```python
from build123d import *

# Parameters (mm, degrees)
BOSS_EXTRUDE1_DEPTH = 11.1125
SKETCH2_R           = 3.96875
BOSS_EXTRUDE2_DEPTH = 9.525
SKETCH4_R           = 3.96875
BOSS_EXTRUDE3_DEPTH = 9.525
FILLET1_R           = 3.175


with BuildPart() as part:
    # Sketch1 → Boss-Extrude1 (new body)
    with BuildSketch(Plane(origin=(0, 0, 0), x_dir=(1, 0, 0), z_dir=(0, 1, 0))):
        with BuildLine():
            Line((-6.133628997, -1.643500936), (-18.005791029, 42.664010964))
            Line((-18.005791029, 42.664010964), (-17.239087405, 42.869448581))
            Line((-17.239087405, 42.869448581), (-5.366925372, -1.438063319))
            ThreePointArc((-5.366925372, -1.438063319), (0.484259096, -5.535106791), (5.535106791, -0.484259096))
            Line((5.535106791, -0.484259096), (9.532985307, 45.211701443))
            Line((9.532985307, 45.211701443), (10.323714849, 45.142521572))
            Line((10.323714849, 45.142521572), (6.325836333, -0.553438966))
            ThreePointArc((6.325836333, -0.553438966), (0.553438966, -6.325836333), (-6.133628997, -1.643500936))
        make_face()
    extrude(amount=BOSS_EXTRUDE1_DEPTH)

    # Sketch2 → Boss-Extrude2 (add)
    with BuildSketch(Plane(origin=(6.325836333, 0, 0.553438966), x_dir=(0.08715574274765789, 0, -0.9961946980917457), z_dir=(0.9961946980917457, 0, 0.08715574274765789))):
        with Locations(Location((39.520511684, 5.55625, 0), (0, 0, 180))):
            Circle(SKETCH2_R)
    extrude(amount=BOSS_EXTRUDE2_DEPTH)

    # Sketch4 → Boss-Extrude3 (add)
    with BuildSketch(Plane(origin=(-6.133628997, 0, 1.643500936), x_dir=(0.2588190451025218, 0, 0.9659258262890681), z_dir=(-0.9659258262890681, 0, 0.2588190451025218))):
        with Locations((-39.520511684, 5.55625)):
            Circle(SKETCH4_R)
    extrude(amount=BOSS_EXTRUDE3_DEPTH)

    # Fillet1
    fillet1_edges = [part.edges().sort_by_distance(p)[0] for p in [
        (19.604929736, 5.55625, -41.940174498),
        (-26.589921674, 5.55625, -37.898648686),
    ]]
    fillet(fillet1_edges, radius=FILLET1_R)


solid = part.part
```
Verification items for the finished model (mm, model axes). A direction names the side the tool comes from. Coordinates: 2 decimals unless noted, no trailing zeros. Order: outer loops, then holes, each group sorted by start corner. A loop starts at its lowest first (then second) coordinate and runs counter-clockwise, first axis right, second up. Notation, with made-up numbers: (48.25, -30) - (82.25, -30) arc R30 cw to (82.25, -6) - close; hole circle Ø3 at (14, 43). An arc over 180 degrees is marked (long way). Return JSON: item names as keys, results as strings.
(1) Go/stop test with flat-tipped pins: pin 1 (1.5 mm diameter, centred on y = 5.5, z = -38.5, fed in from +X); pin 2 (3 mm diameter, centred on x = -2.5, y = 7, fed in from +Z); pin 3 (3 mm diameter, centred on y = 7.5, z = -36.5, fed in from +X). Record where each tip stops, or that it passes through.
Filled sheet:
{"pin 1": "stops at x = 19.34", "pin 2": "stops at z = 6.27", "pin 3": "stops at x = 19.22"}
(2) Access from +Z, -Z, +X, -X, +Y, -Y to the whole of each face (thin tool, end or side, straight path). Record for faces 1 (the cylindrical face through (-18.834, 8.903, -33.659)), 2 (the flat face through (-11.386, 5.478, -21.026)).
Filled sheet:
{"face 1": "none", "face 2": "-Z, +Y, -Y"}
(3) Section check C-C, the plane x = -4.5. Record the cut outline in (y, z).
Filled sheet:
{"outline": "(0, 3.26) - (11.11, 3.26) - (11.11, 4.48) - (0, 4.48) - close"}
(4) Section check A-A, the plane y = 10.5. Record the cut outline in (x, z), and give its area (3 significant figures).
Filled sheet:
{"outline": "(-18.01, -42.66) - (-17.24, -42.87) - (-5.37, 1.44) arc R5.56 cw to (5.54, 0.48) - (9.53, -45.21) - (10.32, -45.14) - (6.33, 0.55) arc R6.35 ccw to (-6.13, 1.64) - close", "area": "86.0 mm^2"}
(5) Thickness scan on line 1 along X through (y, z) = (8.5, -21.5); line 2 along X through (y, z) = (5.5, -5); line 3 along Z through (x, y) = (17, 3.25). Record the ranges inside material, lowest first.
Filled sheet:
{"line 1": "x = -12.33 to -11.51, 7.46 to 8.26", "line 2": "x = -7.91 to -7.09, 6.01 to 6.81", "line 3": "z = -41.35 to -35.22"}
(6) Section check D-D, the plane z = 3. Record the cut outline in (x, y).
Filled sheet:
{"outline": "(-5.6, 0) - (-4.68, 0) - (-4.68, 11.11) - (-5.6, 11.11) - close; (4.68, 0) - (5.6, 0) - (5.6, 11.11) - (4.68, 11.11) - close"}
(7) Section check B-B, the plane z = -6.5. Record the cut outline in (x, y), and give its area (3 significant figures).
Filled sheet:
{"outline": "(-8.32, 0) - (-7.49, 0) - (-7.49, 11.11) - (-8.32, 11.11) - close; (6.15, 0) - (6.94, 0) - (6.94, 11.11) - (6.15, 11.11) - close", "area": "18.0 mm^2"}
(8) Mould release check, pull along X, two halves, no side actions. Record for faces 3 (the flat face through (7.506, 5.478, -22.044)), 4 (the flat face through (-11, 0, -18)), 5 (the flat face through (-25.566, 5.567, -34.076)): pulls with the +X half, pulls with the -X half, needs draft (parallel to the pull), parting line crosses it, or undercut.
Filled sheet:
{"face 3": "undercut", "face 4": "needs draft", "face 5": "pulls with the -X half"}
